from build123d import *

# Parameters (mm, degrees)
SKETCH1_W           = 33.02
SKETCH1_H           = 25.4
SKETCH1_R           = 1.5875
BOSS_EXTRUDE1_DEPTH = 1.5748
SKETCH2_W           = 15.24
SKETCH2_H           = 6.35
BOSS_EXTRUDE2_DEPTH = 7.62
SKETCH3_R           = 2.5
BOSS_EXTRUDE3_DEPTH = 6.35
FILLET1_R           = 1.27


with BuildPart() as part:
    # Sketch1 → Boss-Extrude1 (new body)
    with BuildSketch(Plane(origin=(0, 0, 0), x_dir=(1, 0, 0), z_dir=(0, 1, 0))):
        with Locations((16.51, 12.7)):
            Rectangle(SKETCH1_W, SKETCH1_H)
        with Locations(Location((3.81, 12.7, 0), (0, 0, 270))):
            Circle(SKETCH1_R, mode=Mode.SUBTRACT)
        with Locations(Location((29.21, 12.7, 0), (0, 0, 270))):
            Circle(SKETCH1_R, mode=Mode.SUBTRACT)
    extrude(amount=BOSS_EXTRUDE1_DEPTH)

    # Sketch2 → Boss-Extrude2 (add)
    with BuildSketch(Plane(origin=(0, 1.5748, 0), x_dir=(1, 0, 0), z_dir=(0, 1, 0))):
        with Locations((16.51, 11.43)):
            Rectangle(SKETCH2_W, SKETCH2_H)
    extrude(amount=BOSS_EXTRUDE2_DEPTH)

    # Sketch3 → Boss-Extrude3 (add)
    with BuildSketch(Plane(origin=(0, 1.5748, 0), x_dir=(1, 0, 0), z_dir=(0, 1, 0))):
        with Locations(Location((5.063331186, 20.404812086, 0), (0, 0, 90))):
            Circle(SKETCH3_R)
        with Locations(Location((27.956668814, 20.404812086, 0), (0, 0, 90))):
            Circle(SKETCH3_R)
    extrude(amount=BOSS_EXTRUDE3_DEPTH)

    # Fillet1
    fillet1_edges = [part.edges().sort_by_distance(p)[0] for p in [
        (5.063331186, 7.9248, -17.904812086),
        (27.956668814, 7.9248, -17.904812086),
    ]]
    fillet(fillet1_edges, radius=FILLET1_R)


solid = part.part
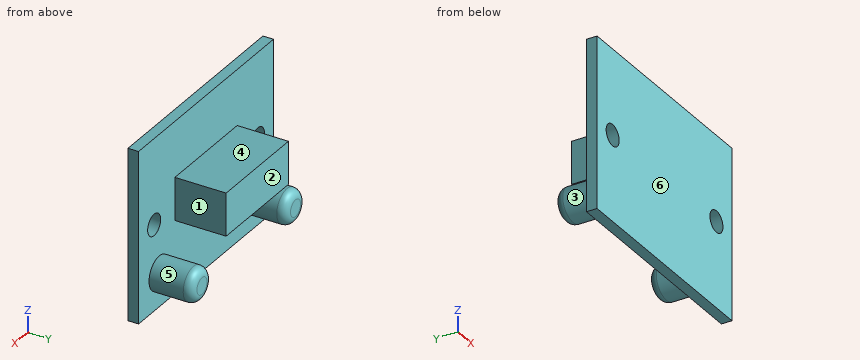
Model file for the job. Use its own axes, mm. Face numbers are marked on the shaded views. A direction names the side the tool comes from. Round coordinates to 2 decimals unless told otherwise and drop trailing zeros. Loops run counter-clockwise (first coordinate to the right, second up) from the corner with the lowest first, then second, coordinate; pieces in that order, holes last. Notation, with made-up numbers: (5.25, -8.75) -> (33.25, -8.75) arc R17 cw to (33.25, -1.75) -> close; hole circle Ø7 at (54, 39). An arc over 180 degrees is marked (long way). Answer as CSV lines item,"result". Start each with the question number.
1) Pin check, flat tips, straight feed: P1, Ø3, axis at y = 5, z = -12.5, coming from the -X side; P2, Ø5, axis at x = 24.5, y = 6.5, coming from the -Z side; P3, Ø1, axis at x = 24.5, y = 3, coming from the +Z side (3 decimals). Stop position of each tip, or through.
2) Slice it at C-C (y = 4.25). List the corners of the cut face in (x, z) (3 decimals), plus the area to 3 significant figures.
3) Probe line 1 along X through (y, z) = (0.95, -12.7); line 2 along X through (y, z) = (6.25, -14.5); line 3 along Z through (x, y) = (20, 8.5) (3 decimals). List the from-to ranges inside material, lowest first.
4) Mould opens along X. For the marked faces 1, 2 and 3 say: +X half, -X half, draft (parallel to the pull), parting line (faces both ways), or undercut.
5) Slice it at A-A (z = -12.7). List the corners of the cut face in (x, y).
6) Slice it at B-B (z = -10). List the corners of the cut face in (x, y), plus the area to 3 significant figures.
7) Slice it at D-D (x = 23). List the corners of the cut face in (y, z) (3 decimals), plus the area to 3 significant figures.
8) Tool access for the marked faces 4, 5 and 6: list every direction of +Z, -Z, +X, -X, +Y, -Y with a clear straight run to the whole face (end or side of a thin tool).
Filled in:
1,P1,"stops at x = 8.89"
1,P2,"stops at z = -22.71"
1,P3,"stops at z = -8.255"
2,outline,"circle Ø5 at (5.063, -20.405); (8.89, -14.605) -> (24.13, -14.605) -> (24.13, -8.255) -> (8.89, -8.255) -> close; circle Ø5 at (27.957, -20.405)"
2,area,"136 mm2"
3,line 1,"x = 0 to 2.22, 5.4 to 27.62, 30.8 to 33.02"
3,line 2,"x = 8.89 to 24.13"
3,line 3,"z = -14.605 to -8.255"
4,face 1,"+X half"
4,face 2,"draft"
4,face 3,"undercut"
5,outline,"(0, 0) -> (2.22, 0) -> (2.22, 1.57) -> (0, 1.57) -> close; (5.4, 0) -> (27.62, 0) -> (27.62, 1.57) -> (24.13, 1.57) -> (24.13, 9.19) -> (8.89, 9.19) -> (8.89, 1.57) -> (5.4, 1.57) -> close; (30.8, 0) -> (33.02, 0) -> (33.02, 1.57) -> (30.8, 1.57) -> close"
6,outline,"(0, 0) -> (33.02, 0) -> (33.02, 1.57) -> (24.13, 1.57) -> (24.13, 9.19) -> (8.89, 9.19) -> (8.89, 1.57) -> (0, 1.57) -> close"
6,area,"168 mm2"
7,outline,"(0, -25.4) -> (1.575, -25.4) -> (1.575, -14.605) -> (9.195, -14.605) -> (9.195, -8.255) -> (1.575, -8.255) -> (1.575, 0) -> (0, 0) -> close"
7,area,"88.4 mm2"
8,face 4,"+Z, +X, -X, +Y"
8,face 5,"+Y"
8,face 6,"+Z, -Z, +X, -X, -Y"
